Input: dimensioned drawing with shaded views. Units: mm. Origin: part minimum x, y, z. A direction names the side the tool comes from. Give positions to 0.01 mm unless a question says otherwise; leave off trailing zeros. Write each loop counter-clockwise with the first axis right and the second up, starting at its lowest first coordinate (ties: lowest second). Pieces come first, ordered by that corner, then holes.
Q1. Pin query (flat end, axial travel): pin 1 Ø4 at (x, y) = (18.5, 25) entering from +Z; pin 2 Ø3.5 at (x, y) = (25.4, 22.225) entering from +Z. Return the tip coordinate at first contact, or that it passes through.
Q2. Line query: line 1 (X direction, y = 24.5, z = 12.5); line 2 (Y direction, x = 38.1, z = 4); line 3 (Y direction, x = 36, z = 22) (3 decimals). Output: solid intervals per line, ascending.
Q3. Section C-C (y = 17.5). Return the cut outline in (x, z), plus the area to 3 significant figures.
Q4. Section D-D (z = 12.7). Return the cut outline in (x, y) (3 decimals), plus the area to 3 significant figures.
Q5. Reachability of the marked faces 4 and 5 from +Z, -Z, +X, -X, +Y, -Y: full face, straight path, thin tool, end or side. Return the list, or none.
Q6. Section B-B (x = 12.7). Return the cut outline in (y, z) (3 decimals), plus the area to 3 significant figures.
Q7. Mould query, pull axis Y, two halves, no side actions, for the marked faces 1, 2 and 3. Classes: +Y half, -Y half, draft (parallel to the pull), parting line (faces both ways), or undercut.
Q8. Section A-A (z = 22.5). Return the cut outline in (x, y) (3 decimals).
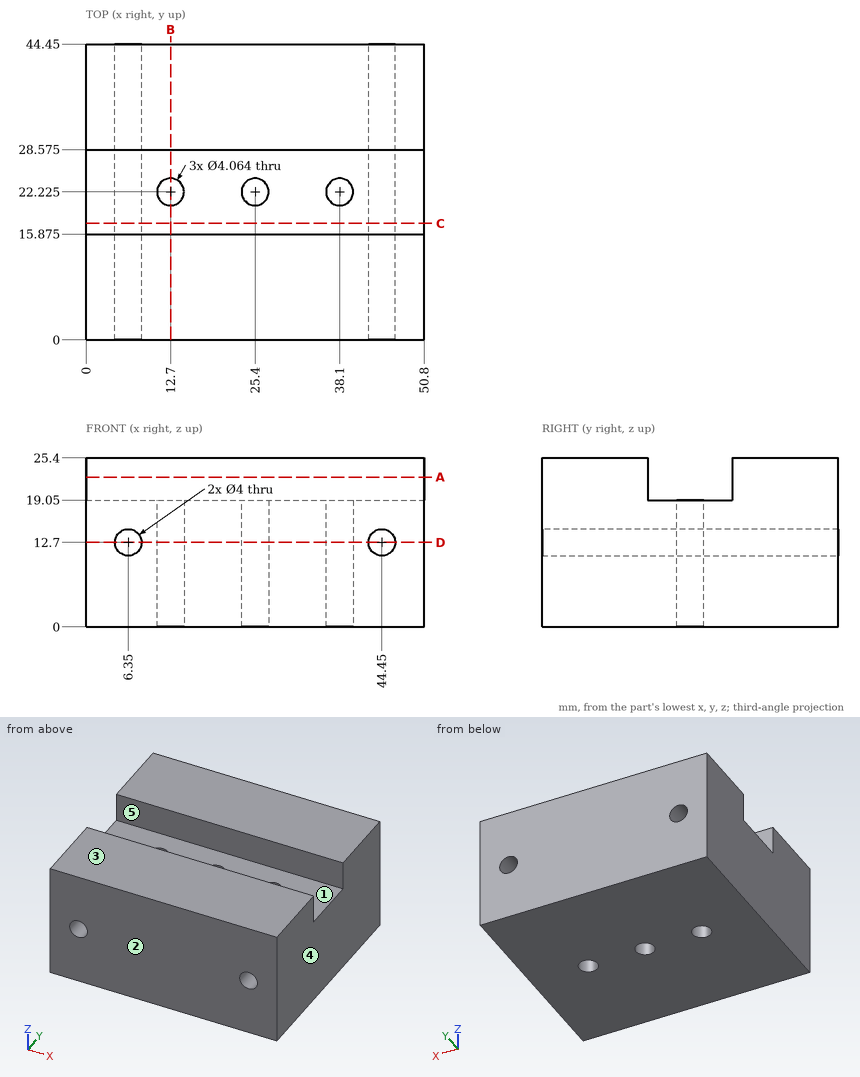
Computed:
1. pin 1: stops at z = 19.05
1. pin 2: passes through
2. line 1: x = 0 to 4.36, 8.34 to 42.46, 46.44 to 50.8
2. line 2: y = 0 to 20.19, 24.26 to 44.45
2. line 3: y = 0 to 15.875, 28.575 to 44.45
3. outline: (0, 0) - (50.8, 0) - (50.8, 19.05) - (0, 19.05) - close; hole circle Ø4 at (6.35, 12.7); hole circle Ø4 at (44.45, 12.7)
3. area: 943 mm2
4. outline: (0, 0) - (4.35, 0) - (4.35, 44.45) - (0, 44.45) - close; (8.35, 0) - (42.45, 0) - (42.45, 44.45) - (8.35, 44.45) - close; (46.45, 0) - (50.8, 0) - (50.8, 44.45) - (46.45, 44.45) - close; hole circle Ø4.064 at (12.7, 22.225); hole circle Ø4.064 at (25.4, 22.225); hole circle Ø4.064 at (38.1, 22.225)
4. area: 1,860 mm2
5. face 4: +Z, -Z, +X, +Y, -Y
5. face 5: +Z, +X, -X
6. outline: (0, 0) - (20.193, 0) - (20.193, 19.05) - (15.875, 19.05) - (15.875, 25.4) - (0, 25.4) - close; (24.257, 0) - (44.45, 0) - (44.45, 25.4) - (28.575, 25.4) - (28.575, 19.05) - (24.257, 19.05) - close
6. area: 971 mm2
7. face 1: undercut
7. face 2: -Y half
7. face 3: draft
8. outline: (0, 0) - (50.8, 0) - (50.8, 15.875) - (0, 15.875) - close; (0, 28.575) - (50.8, 28.575) - (50.8, 44.45) - (0, 44.45) - close
